Geometry check sheet. Reference: the model listing, model coordinates, mm. Round coordinates to 2 decimals unless told otherwise and drop trailing zeros. Loops run counter-clockwise (first coordinate to the right, second up) from the corner with the lowest first, then second, coordinate; pieces in that order, holes last. Notation, with made-up numbers: (-34.5, 69.25) -> (18.5, 69.25) arc R31 ccw to (18.5, 97.25) -> close; hole circle Ø5 at (-32.5, -29). An arc over 180 degrees is marked (long way). Use a Markdown table: item, result. Add a question column.
Q1. Release check for a two-part mould opening along Z. For faces 1 (the face through (0, 3, -1)), 2 (the face through (-11, 2, 68)), 3 (the face through (-5.54, 1.52, -40.06)), 4 (the face through (-10, 2, -69)) record: released by +Z, released by -Z, zero draft, split by the parting line, or undercut.
Q2. Sectioned sample at C-C, the plane y = 2.25. Give the number of separate pieces and of enclosed holes in the cut face, then the cut area to 3 significant figures.
Q3. Material ranges on L1, parallel to Z at x = 5, y = 2.3; L2, parallel to X at y = 1.05, z = 42.5; L3, parallel to Z at x = -5.5, y = 0.55, recorded low to high.
Q4. Gauge pin test, flat ends, axial feed: P1, Ø3, axis at x = 5, z = 62.5, coming from the -Y side; P2, Ø12, axis at x = 8, z = 38.5, coming from the -Y side. Record the tip position at first contact, or that the pin passes through.
Q5. Sectioned sample at B-B, the plane z = -42.5. Enter the section's corners in (x, y).
Q6. Sectioned sample at A-A, the plane x = 5. Enter the section's corners in (y, z), then the cut area to 3 significant figures.
Q7. Sectioned sample at D-D, the plane x = -5.25. Enter the section's corners in (y, z).
```python
from build123d import *

# Parameters (mm, degrees)
SKETCH_1_R      = 2.5
EXTRUDE_1_DEPTH = 3


with BuildPart() as part:
    # 草圖1 → 填料-伸長1 (new body)
    with BuildSketch(Plane(origin=(0, 3, 0), x_dir=(1, 0, 0), z_dir=(0, 1, 0))):
        Polygon((-12, 67), (-12, -67), (-9, -70), (9, -70), (12, -67), (12, 67), (9, 70), (-9, 70), align=None)
        with Locations((-5, 62.5)):
            Circle(SKETCH_1_R, mode=Mode.SUBTRACT)
        with Locations((5, 62.5)):
            Circle(SKETCH_1_R, mode=Mode.SUBTRACT)
        with Locations((5, 42.5)):
            Circle(SKETCH_1_R, mode=Mode.SUBTRACT)
        with Locations((-5, 42.5)):
            Circle(SKETCH_1_R, mode=Mode.SUBTRACT)
        with Locations((5, -42.5)):
            Circle(SKETCH_1_R, mode=Mode.SUBTRACT)
        with Locations((-5, -42.5)):
            Circle(SKETCH_1_R, mode=Mode.SUBTRACT)
        with Locations((5, -62.5)):
            Circle(SKETCH_1_R, mode=Mode.SUBTRACT)
        with Locations((-5, -62.5)):
            Circle(SKETCH_1_R, mode=Mode.SUBTRACT)
    extrude(amount=-EXTRUDE_1_DEPTH)


solid = part.part
```
Values:
| question | item | result |
|---|---|---|
| 1 | face 1 | zero draft |
| 1 | face 2 | released by +Z |
| 1 | face 3 | undercut |
| 1 | face 4 | released by -Z |
| 2 | separate pieces | 1 |
| 2 | enclosed holes | 8 |
| 2 | area | 3,180 mm^2 |
| 3 | L1 | -70 to -65, -60 to -45, -40 to 40, 45 to 60, 65 to 70 |
| 3 | L2 | -12 to -7.5, -2.5 to 2.5, 7.5 to 12 |
| 3 | L3 | -70 to -64.95, -60.05 to -44.95, -40.05 to 40.05, 44.95 to 60.05, 64.95 to 70 |
| 4 | P1 | through |
| 4 | P2 | y = 0 |
| 5 | outline | (-12, 0) -> (-7.5, 0) -> (-7.5, 3) -> (-12, 3) -> close; (-2.5, 0) -> (2.5, 0) -> (2.5, 3) -> (-2.5, 3) -> close; (7.5, 0) -> (12, 0) -> (12, 3) -> (7.5, 3) -> close |
| 6 | outline | (0, -70) -> (3, -70) -> (3, -65) -> (0, -65) -> close; (0, -60) -> (3, -60) -> (3, -45) -> (0, -45) -> close; (0, -40) -> (3, -40) -> (3, 40) -> (0, 40) -> close; (0, 45) -> (3, 45) -> (3, 60) -> (0, 60) -> close; (0, 65) -> (3, 65) -> (3, 70) -> (0, 70) -> close |
| 6 | area | 360 mm^2 |
| 7 | outline | (0, -70) -> (3, -70) -> (3, -64.99) -> (0, -64.99) -> close; (0, -60.01) -> (3, -60.01) -> (3, -44.99) -> (0, -44.99) -> close; (0, -40.01) -> (3, -40.01) -> (3, 40.01) -> (0, 40.01) -> close; (0, 44.99) -> (3, 44.99) -> (3, 60.01) -> (0, 60.01) -> close; (0, 64.99) -> (3, 64.99) -> (3, 70) -> (0, 70) -> close |
